Design review of the part built by this model. Coordinates are the model's own, in mm. A direction names the side the tool comes from. Coordinates: 2 decimals unless noted, no trailing zeros. Loops run counter-clockwise (first coordinate to the right, second up) from the corner with the lowest first, then second, coordinate; pieces in that order, holes last. Notation, with made-up numbers: (3, 63.25) - (13, 63.25) arc R23 ccw to (13, 92.25) - close; hole circle Ø10 at (-8.75, -14.5). An arc over 180 degrees is marked (long way). Return JSON: item names as keys, results as strings. Group by question number.
from build123d import *

# Parameters (mm, degrees)
BOSS_EXTRUDE1_DEPTH = 10
CUT_EXTRUDE1_DEPTH  = 12
CUT_EXTRUDE2_DEPTH  = 1.6
FILLET1_R           = 2


with BuildPart() as part:
    # Sketch1 → Boss-Extrude1 (new body)
    with BuildSketch(Plane(origin=(0, 0, 0), x_dir=(0, 0, -1), z_dir=(1, 0, 0))):
        Polygon((102.124722519, 158.335097964), (93.821109228, 161.348394189), (97.419958261, 171.26559065), (106.408476892, 168.00374929), (104.484281292, 160.826776001), align=None)
    extrude(amount=BOSS_EXTRUDE1_DEPTH)

    # Sketch2 → Cut-Extrude1 (cut)
    with BuildSketch(Plane(origin=(0, 96.421451451, -272.737546345), x_dir=(1, 0, 0), z_dir=(0, -0.940018622, 0.341123131))):
        Polygon((2.031147255, 188.996331096), (0.775279506, 185.892119516), (2.835671718, 183.252400352), (6.151931679, 183.716892768), (7.407799428, 186.821104348), (5.347407216, 189.460823512), align=None)
    extrude(amount=-CUT_EXTRUDE1_DEPTH, mode=Mode.SUBTRACT)

    # Sketch3 → Cut-Extrude2 (cut)
    with BuildSketch(Plane(origin=(0, 172.657963315, -62.655806689), x_dir=(1, 0, 0), z_dir=(0, -0.940018622, 0.341123131))):
        Polygon((0, -33.153920374), (8.2, -33.153920374), (8.2, -42.73147424), (8.2, -44.631348282), (0, -44.631348282), (0, -42.73147424), align=None)
    extrude(amount=-CUT_EXTRUDE2_DEPTH, mode=Mode.SUBTRACT)

    # Fillet1
    fillet1_edges = [part.edges().sort_by_distance(p)[0] for p in [
        (0, 164.415262646, -105.446379092),
    ]]
    fillet(fillet1_edges, radius=FILLET1_R)


solid = part.part
Item 1: Add section D-D (x = 7.75). State the section outline as (y, z) points, then the cut area to 3 significant figures.
Item 2: Draft analysis for pull direction X (two halves, no side actions). For faces 1 (the face through (10, 165, -100)), 2 (the face through (5.98, 160.53, -100.77)), 3 (the face through (1.79, 165.04, -101.27)), state which applies: pulls with the +X half, pulls with the -X half, needs draft (parallel to the pull), parting line crosses it, or undercut.
Item 3: Add section A-A (x = 1.25). State the section outline as (y, z) points, then the cut area to 3 significant figures.
Item 4: For faces 4 (the face through (4.47, 164.66, -102.31)), 5 (the face through (4, 167, -97)), 6 (the face through (6.771, 165.265, -100.653)), list the 3-axis set-ups (+Z, -Z, +X, -X, +Y, -Y) from which the entire face can be reached by the end or side of a thin tool; tool diameter is ignored.
Item 5: To check wall thickness, follow line 1 (Z direction, x = 5.25, y = 163.25); line 2 (X direction, y = 161, z = -99); line 3 (X direction, y = 162, z = -100). State the ranges of each line that lie inside material, in increasing order. Write a range as from..to.
Item 6: Add section C-C (y = 169.5). State the section outline as (x, z) points.
Item 7: Add section B-B (z = -99.25). State the section outline as (x, y) points, then the cut area to 3 significant figures.
Item 8: For P1, Ø4, axis at x = 8, y = 167.5, coming from the +Z side; P2, Ø6, axis at x = 1, z = -101.5, coming from the -Y side, all flat-tipped, find the tip position at first contact; note any pin that passes through.
Answers below:
{
 "1": {"outline": "(159.6, -103.32) - (160.83, -104.48) - (168, -106.41) - (171.27, -97.42) - (162.85, -94.37) - close", "area": "88.4 mm^2"},
 "2": {"face 1": "pulls with the +X half", "face 2": "needs draft", "face 3": "undercut"},
 "3": {"outline": "(159.6, -103.32) - (160.6, -104.27) - (168.05, -106.27) - (169.54, -102.17) - (161.13, -99.11) - close; (161.74, -97.44) - (170.15, -100.49) - (171.27, -97.42) - (162.85, -94.37) - close", "area": "71.4 mm^2"},
 "4": {"face 4": "+Y", "face 5": "-Y", "face 6": "none"},
 "5": {"line 1": "z = -105.13..-101.68, -95.45..-94.51", "line 2": "x = 8.2..10", "line 3": "x = 0..1.67, 6.57..10"},
 "6": {"outline": "(0, -102.29) - (1.35, -102.29) - (0.78, -101.5) - (2.03, -98.2) - (5.35, -97.71) - (7.41, -100.52) - (6.73, -102.29) - (10, -102.29) - (10, -96.78) - (0, -96.78) - close"},
 "7": {"outline": "(0, 161.08) - (1.36, 161.08) - (0.78, 163.29) - (1.78, 170.6) - (0, 170.6) - close; (6.19, 170.6) - (7.41, 166.01) - (6.73, 161.08) - (8.2, 161.08) - (8.2, 159.38) - (10, 159.38) - (10, 170.6) - close", "area": "43.9 mm^2"},
 "8": {"P1": "stops at z = -95.33", "P2": "stops at y = 159.6"}
}
